Autodesk Inventor part; units mm, degrees
ref_plane "YZ Plane" through (0, 0, 0) normal (1, 0, 0) x (0, 1, 0)
ref_plane "XZ Plane" through (0, 0, 0) normal (0, 1, 0) x (-1, 0, 0)
ref_plane "XY Plane" through (0, 0, 0) normal (0, 0, 1) x (1, 0, 0)
sketch "Sketch1" plane through (0, 0, 0) normal (0, 0, 1) x (1, 0, 0)
  line L0 (0, 0) -> (50, 0)
  line L1 (50, 0) -> (50, 10)
  line L2 (50, 10) -> (0, 10)
  line L3 (0, 10) -> (0, 0)
  circle A0 centre (4, 5) radius 1.5
  circle A1 centre (46, 5) radius 1.5
  point P0 (0, 5)
  dimension "d0" = 50
  dimension "d1" = 10
  dimension "d22" = 3
  dimension "d23" = 3
  dimension "d24" = 4
  dimension "d25" = 4
extrude "Extrusion1" add sketch "Sketch1" along normal blind 5
sketch "Sketch2" plane through (0, 0, 5) normal (0, 0, 1) x (1, 0, 0)
  line L0 (50, 10) -> (0, 10)
  line L1 (0, 0) -> (50, 0)
  line L2 (12.5, 10) -> (37.5, 10)
  line L3 (37.5, 10) -> (37.5, 6)
  line L4 (37.5, 6) -> (12.5, 6)
  line L5 (12.5, 6) -> (12.5, 10)
  line L6 (12.5, 0) -> (37.5, 0)
  line L7 (37.5, 0) -> (37.5, 4)
  line L8 (37.5, 4) -> (12.5, 4)
  line L9 (12.5, 4) -> (12.5, 0)
  point P0 (25, 10)
  point P1 (25, 10)
  point P2 (25, 0)
  point P3 (25, 0)
  dimension "d14" = 25
  dimension "d15" = 25
  dimension "d31" = 2
  dimension "d32" = 4
  dimension "d33" = 4
extrude "Extrusion2" add sketch "Sketch2" along normal blind 13
fillet "Fillet1" radius 1 2 edges at (25, 6, 18) (25, 4, 18)
sketch "Sketch3" plane through (0, 0, 5) normal (0, 0, 1) x (1, 0, 0)
  circle A0 centre (4, 5) radius 1.5
  circle A1 centre (46, 5) radius 1.5
  line L0 (6.75, 6.5877) -> (6.75, 3.4123)
  line L1 (6.75, 3.4123) -> (4, 1.8246)
  line L2 (4, 1.8246) -> (1.25, 3.4123)
  line L3 (1.25, 3.4123) -> (1.25, 6.5877)
  line L4 (1.25, 6.5877) -> (4, 8.1754)
  line L5 (4, 8.1754) -> (6.75, 6.5877)
  line L6 (43.25, 6.5877) -> (46, 8.1754)
  line L7 (46, 8.1754) -> (48.75, 6.5877)
  line L8 (48.75, 6.5877) -> (48.75, 3.4123)
  line L9 (48.75, 3.4123) -> (46, 1.8246)
  line L10 (46, 1.8246) -> (43.25, 3.4123)
  line L11 (43.25, 3.4123) -> (43.25, 6.5877)
  point P0 (0, 0)
  dimension "d39" = 5.5
  dimension "d40" = 5.5
extrude "Extrusion3" cut sketch "Sketch3" against normal blind 3
sketch "Sketch4" plane through (0, 0, 5) normal (0, 0, 1) x (1, 0, 0)
  line L0 (12.5, 6) -> (12.5, 10)
  line L1 (37.5, 4) -> (37.5, 0)
  line L2 (12.5, 6) -> (37.5, 6)
  line L3 (37.5, 6) -> (37.5, 4)
  line L4 (37.5, 4) -> (12.5, 4)
  line L5 (12.5, 4) -> (12.5, 6)
  point P0 (0, 0)
extrude "Extrusion4" add sketch "Sketch4" along normal blind 4
equation "\"d15\" = d14"
equation "\"d32\" = d33"
equation "\"d40\" = d39"
properties part number "GT2 grip"
Here's how the part is built. I have some questions about the finished solid (model axes, mm). A direction names the side the tool comes from. Round coordinates to 2 decimals unless told otherwise and drop trailing zeros. Loops run counter-clockwise (first coordinate to the right, second up) from the corner with the lowest first, then second, coordinate; pieces in that order, holes last. Notation, with made-up numbers: (-10.75, 75) - (27.25, 75) arc R18 cw to (27.25, 98) - close; hole circle Ø5 at (-22, 8). An arc over 180 degrees is marked (long way). One line per question, with ' | ' between items. Start each with the question number.
Q1. I want a section at B-B (z = 14). Write out the boundary of the cut face in (x, y), then the cut area to 3 significant figures.
Q2. I want a section at D-D (z = 6.5). Write out the boundary of the cut face in (x, y).
Q3. I want a section at A-A (y = 5). Write out the boundary of the cut face in (x, z).
Q4. I want a section at C-C (x = 23.5). Write out the boundary of the cut face in (y, z), then the cut area to 3 significant figures.
Q5. We'd pull the mould along Y, two halves only. Please class faces 5 (the flat face through (43.25, 5, 4)), 6 (the flat face through (50, 5, 2)): +Y half, -Y half, draft (parallel to the pull), parting line (faces both ways), or undercut.
Q6. Please list where these lines run through material, in increasing order: line 1 (Y direction, x = 4, z = 0.75); line 2 (Y direction, x = 28, z = 11.75); line 3 (X direction, y = 2, z = 12.25). Write a range as [from, to].
Q7. Will these pins go through, and if not, where does the flat tip stop? pin 1 (5 mm diameter, centred on x = 4, y = 5, fed in from +Z); pin 2 (2 mm diameter, centred on x = 15.5, y = 5.5, fed in from +Z); pin 3 (5 mm diameter, centred on y = 4, z = 8.5, fed in from +X); pin 4 (2.5 mm diameter, centred on x = 46, y = 5, fed in from -Z).
Q8. For faces 1 (the flat face through (8, 5, 5)), 2 (the flat face through (5.394, 2.63, 3.521)), 3 (the flat face through (25, 6, 13)), 4 (the flat face through (0, 5, 2)), which set-ups out of +Z, -Z, +X, -X, +Y, -Y let a thin tool reach every point of the face, with its end or its side?
Response values:
1) outline: (12.5, 0) - (37.5, 0) - (37.5, 4) - (12.5, 4) - close; (12.5, 6) - (37.5, 6) - (37.5, 10) - (12.5, 10) - close | area: 200 mm²
2) outline: (12.5, 0) - (37.5, 0) - (37.5, 10) - (12.5, 10) - close
3) outline: (0, 0) - (2.5, 0) - (2.5, 2) - (1.25, 2) - (1.25, 5) - (0, 5) - close; (5.5, 0) - (44.5, 0) - (44.5, 2) - (43.25, 2) - (43.25, 5) - (37.5, 5) - (37.5, 9) - (12.5, 9) - (12.5, 5) - (6.75, 5) - (6.75, 2) - (5.5, 2) - close; (47.5, 0) - (50, 0) - (50, 5) - (48.75, 5) - (48.75, 2) - (47.5, 2) - close
4) outline: (0, 0) - (10, 0) - (10, 18) - (7, 18) arc R1 ccw to (6, 17) - (6, 9) - (4, 9) - (4, 17) arc R1 ccw to (3, 18) - (0, 18) - close | area: 162 mm²
5) face 5: undercut | face 6: draft
6) line 1: y = [0, 3.5], [6.5, 10] | line 2: y = [0, 4], [6, 10] | line 3: x = [12.5, 37.5]
7) pin 1: stops at z = 2 | pin 2: stops at z = 17.87 | pin 3: stops at x = 37.5 | pin 4: passes through
8) face 1: +Z, -X, +Y, -Y | face 2: +Z | face 3: +Z, +X, -X | face 4: +Z, -Z, -X, +Y, -Y
